Drawing for the job (mm, zero at the part's lowest x, y, z). A direction names the side the tool comes from. Round coordinates to 2 decimals unless told otherwise and drop trailing zeros. Write each loop counter-clockwise with the first axis right and the second up, starting at its lowest first coordinate (ties: lowest second). Pieces come first, ordered by that corner, then holes.
Item 1: 3-axis set-ups, long thin cutter, end or side, ignore diameter. For the marked faces 1, 2 and 3: which of +Z, -Z, +X, -X, +Y, -Y reach the whole face in a straight line?
Item 2: Band-saw the part on B-B, the plane y = 21.75. Write the cut outline in (x, z), then the cut area to 3 significant figures.
Item 3: Band-saw the part on D-D, the plane y = 6.25. Write the cut outline in (x, z).
Item 4: Band-saw the part on C-C, the plane x = 2.5. Write the cut outline in (y, z), then the cut area to 3 significant figures.
Item 5: Wall check: probe 1 along Y at (x, z) = (12.95, 10.75); probe 2 along Z at (x, y) = (13, 2.25); probe 3 along X at (y, z) = (19.25, 1). Give the ranges that are in metal, low to high.
Item 6: Band-saw the part on A-A, the plane x = 12.95. Write the cut outline in (y, z).
Item 7: Drop flat-ended pins along their axis: pin 1 Ø3 at (x, z) = (11.5, 8) entering from +Y; pin 2 Ø8 at (x, y) = (9.5, 7) entering from -Z; pin 3 Ø1.5 at (x, z) = (2, 3.5) entering from -Y; pin 4 Ø5.5 at (x, y) = (12.95, 6.25) entering from +Z. Give the stop position or say it passes through.
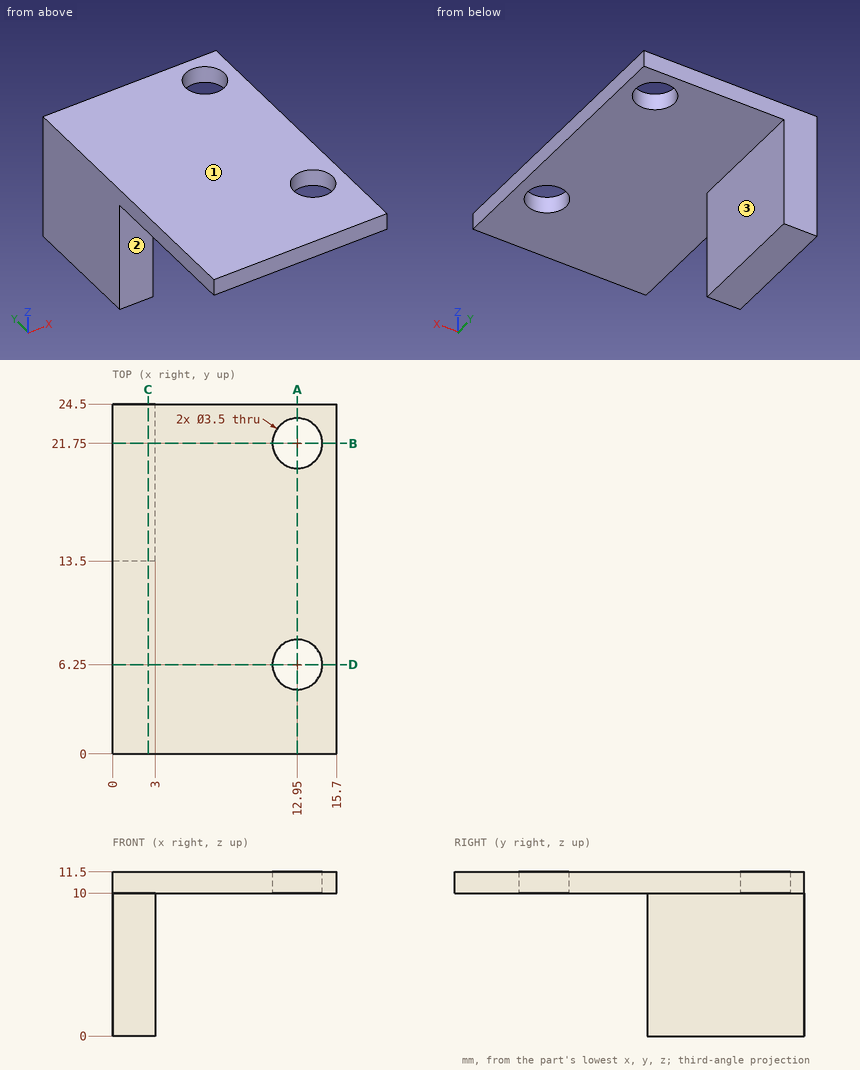
Results:
1. face 1: +Z, +X, -X, +Y, -Y
1. face 2: -Z, +X, -X, -Y
1. face 3: -Z, +X, +Y, -Y
2. outline: (0, 0) - (3, 0) - (3, 10) - (11.2, 10) - (11.2, 11.5) - (0, 11.5) - close; (14.7, 10) - (15.7, 10) - (15.7, 11.5) - (14.7, 11.5) - close
2. area: 48.3 mm2
3. outline: (0, 10) - (11.2, 10) - (11.2, 11.5) - (0, 11.5) - close; (14.7, 10) - (15.7, 10) - (15.7, 11.5) - (14.7, 11.5) - close
4. outline: (0, 10) - (13.5, 10) - (13.5, 0) - (24.5, 0) - (24.5, 11.5) - (0, 11.5) - close
4. area: 147 mm2
5. probe 1: y = 0 to 4.5, 8 to 20, 23.5 to 24.5
5. probe 2: z = 10 to 11.5
5. probe 3: x = 0 to 3
6. outline: (0, 10) - (4.5, 10) - (4.5, 11.5) - (0, 11.5) - close; (8, 10) - (20, 10) - (20, 11.5) - (8, 11.5) - close; (23.5, 10) - (24.5, 10) - (24.5, 11.5) - (23.5, 11.5) - close
7. pin 1: passes through
7. pin 2: stops at z = 10
7. pin 3: stops at y = 13.5
7. pin 4: stops at z = 11.5
